```python
from build123d import *

# Parameters (mm, degrees)
SKETCH_1_R          = 1.6
EXTRUDE_1_DEPTH     = 8
EXTRUDE_1_2_DEPTH   = 8
EXTRUDE_1_3_DEPTH   = 8
EXTRUDE_1_4_DEPTH   = 8
SKETCH_2_W          = 109.546924753
SKETCH_2_H          = 70.491732923
EXTRUDE_2_DEPTH     = 2
SKETCH_3_W          = 105.546924753
SKETCH_3_H          = 66.491732923
CUT_EXTRUDE_1_DEPTH = 0.5


with BuildPart() as part:
    # Sketch 1 → Extrude 1 (new body)
    with BuildSketch(Plane.XY):
        with Locations((320.970675526, 77.650698191)):
            Circle(SKETCH_1_R)
    extrude(amount=EXTRUDE_1_DEPTH)



with BuildPart() as body_2:
    # Sketch 1 → Extrude 1 2 (new body)
    with BuildSketch(Plane.XY):
        with Locations(Location((320.970675526, 13.440898947, 0), (0, 0, 180))):
            Circle(SKETCH_1_R)
    extrude(amount=EXTRUDE_1_2_DEPTH)


with BuildPart() as body_3:
    # Sketch 1 → Extrude 1 3 (new body)
    with BuildSketch(Plane.XY):
        with Locations((217.817076829, 13.440898947)):
            Circle(SKETCH_1_R)
    extrude(amount=EXTRUDE_1_3_DEPTH)


with BuildPart() as body_4:
    # Sketch 1 → Extrude 1 4 (new body)
    with BuildSketch(Plane.XY):
        with Locations(Location((217.817076829, 77.650698191, 0), (0, 0, 180))):
            Circle(SKETCH_1_R)
    extrude(amount=EXTRUDE_1_4_DEPTH)


with BuildPart() as part_1:
    add(part.part)

    add(body_2.part)  # Extrude 2 merges body 2

    add(body_3.part)  # Extrude 2 merges body 3

    add(body_4.part)  # Extrude 2 merges body 4
    # Sketch 2 → Extrude 2 (add)
    with BuildSketch(Plane.XY.offset(8)):
        with Locations((269.393876178, 45.545798569)):
            Rectangle(SKETCH_2_W, SKETCH_2_H)
    extrude(amount=EXTRUDE_2_DEPTH)

    # Sketch 3 → Cut-Extrude 1 (cut)
    with BuildSketch(Plane.XY.offset(10)):
        with Locations((269.393876178, 45.545798569)):
            Rectangle(SKETCH_3_W, SKETCH_3_H)
    extrude(amount=-CUT_EXTRUDE_1_DEPTH, mode=Mode.SUBTRACT)


solid = part_1.part
```
Part model, mm, in its own coordinate system. A direction names the side the tool comes from. Round coordinates to 2 decimals unless told otherwise and drop trailing zeros. Loops run counter-clockwise (first coordinate to the right, second up) from the corner with the lowest first, then second, coordinate; pieces in that order, holes last.
Item 1: Cut at C-C, the plane z = 2.5. Give the cut face in (x, y).
Item 2: Drop flat-ended pins along their axis: P1, Ø12, axis at x = 262, y = 20, coming from the -Z side; P2, Ø1, axis at x = 272.5, y = 39, coming from the +Z side; P3, Ø4, axis at y = 70.5, z = 5, coming from the +X side. Give the stop position or say it passes through.
Item 3: Cut at A-A, the plane x = 273.5. Give the cut face in (y, z).
Item 4: Drill centre line: line 1 (Z direction, x = 272, y = 27.5). Where is it in solid material? Low to high.
Item 5: 3-axis set-ups, long thin cutter, end or side, ignore diameter. For faces 1 (the face through (214.62, 45, 9)), 2 (the face through (269, 46, 9.5)), 3 (the face through (216.547, 12.467, 3.944)): which of +Z, -Z, +X, -X, +Y, -Y reach the whole face in a straight line?
Item 6: Cut at B-B, the plane y = 23. Give the cut face in (x, z).
A:
1. outline: circle Ø3.2 at (217.82, 13.44); circle Ø3.2 at (217.82, 77.65); circle Ø3.2 at (320.97, 13.44); circle Ø3.2 at (320.97, 77.65)
2. P1: stops at z = 8
2. P2: stops at z = 9.5
2. P3: passes through
3. outline: (10.3, 8) - (80.79, 8) - (80.79, 10) - (78.79, 10) - (78.79, 9.5) - (12.3, 9.5) - (12.3, 10) - (10.3, 10) - close
4. line 1: z = 8 to 9.5
5. face 1: +Z, -Z, -X, +Y, -Y
5. face 2: +Z
5. face 3: -Z
6. outline: (214.62, 8) - (324.17, 8) - (324.17, 10) - (322.17, 10) - (322.17, 9.5) - (216.62, 9.5) - (216.62, 10) - (214.62, 10) - close
